```python
from build123d import *

# Parameters (mm, degrees)
BOSS_EXTRU_1_DEPTH      = 15
ESQUISSE3_W             = 30
ESQUISSE3_H             = 15
ENL_V_MAT_EXTRU_1_DEPTH = 15


with BuildPart() as part:
    # Esquisse2 → Boss.-Extru.1 (new body)
    with BuildSketch(Plane.XY):
        with BuildLine():
            Line((-120, 0), (120, 0))
            Line((120, 0), (120, 15))
            Line((120, 15), (120, 55.414518843))
            Line((120, 55.414518843), (120, 75.414518843))
            Line((120, 75.414518843), (120, 90))
            ThreePointArc((120, 90), (117.071067812, 97.071067812), (110, 100))
            Line((110, 100), (-110, 100))
            ThreePointArc((-110, 100), (-117.071067812, 97.071067812), (-120, 90))
            Line((-120, 90), (-120, 75.414518843))
            Line((-120, 75.414518843), (-120, 55.414518843))
            Line((-120, 55.414518843), (-120, 15))
            Line((-120, 15), (-120, 0))
        make_face()
    extrude(amount=BOSS_EXTRU_1_DEPTH)

    # Esquisse3 → Enlèv. mat.-Extru.1 (cut)
    with BuildSketch(Plane.XY.offset(15)):
        with Locations((-105, 7.5)):
            Rectangle(ESQUISSE3_W, ESQUISSE3_H)
        Polygon((-5, 31.515847226), (-5, 0), (5, 0), (5, 31.515847226), (12.5, 31.515847226), (12.5, 41.515847226), (5, 41.515847226), (5, 50), (-5, 50), (-5, 41.515847226), (-12.5, 41.515847226), (-12.5, 31.515847226), align=None)
        with Locations((105, 7.5)):
            Rectangle(ESQUISSE3_W, ESQUISSE3_H)
    extrude(amount=-ENL_V_MAT_EXTRU_1_DEPTH, mode=Mode.SUBTRACT)


solid = part.part
```
Input: part model. Units: mm. Frame: model coordinates. A direction names the side the tool comes from. Round coordinates to 2 decimals unless told otherwise and drop trailing zeros. Loops run counter-clockwise (first coordinate to the right, second up) from the corner with the lowest first, then second, coordinate; pieces in that order, holes last. Notation, with made-up numbers: M 56,-14.5 L 98,-14.5 A17 cw 98,1.5 Z; hole C 17,25.25 d6. An arc over 180 degrees is marked long. Answer in a Markdown table with one row per item. Add a question column.
1. Mould query, pull axis X, two halves, no side actions, for faces 1 (the face through (-90, 7, 8)), 2 (the face through (-5, 46, 8)), 3 (the face through (117.15, 96.99, 7.4)). Classes: released by +X, released by -X, zero draft, split by the parting line, or undercut.
2. Section A-A (z = 12). Output: boundary loops of the cut face in (x, y).
3. Set-up query: faces 4 (the face through (-12.5, 37, 8)), 5 (the face through (105, 15, 8)), 6 (the face through (5, 16, 8)), 7 (the face through (-105, 15, 8)). Return all of +Z, -Z, +X, -X, +Y, -Y with unobstructed straight access to the full face (end or side cutting, diameter ignored); none if empty.
4. Section B-B (x = -96). Output: boundary loops of the cut face in (y, z).
5. Contact query for flat-ended pins moving along their axis: pin 1 (3 mm diameter, centred on x = -2, z = 4.5, fed in from -Y); pin 2 (7.5 mm diameter, centred on x = 103, z = 9, fed in from -Y). Output: stop coordinate, or through.
6. Ray query, probe 1 along X at (y, z) = (17, 7.25); probe 2 along X at (y, z) = (6.5, 4.75); probe 3 along Y at (x, z) = (3, 1). Return the intervals inside material, ascending.
Values follow:
| question | item | result |
|---|---|---|
| 1 | face 1 | released by -X |
| 1 | face 2 | undercut |
| 1 | face 3 | released by +X |
| 2 | outline | M -120,15 L -90,15 L -90,0 L -5,0 L -5,31.52 L -12.5,31.52 L -12.5,41.52 L -5,41.52 L -5,50 L 5,50 L 5,41.52 L 12.5,41.52 L 12.5,31.52 L 5,31.52 L 5,0 L 90,0 L 90,15 L 120,15 L 120,90 A10 ccw 110,100 L -110,100 A10 ccw -120,90 Z |
| 3 | face 4 | +Z, -Z |
| 3 | face 5 | +Z, -Z, +X, -Y |
| 3 | face 6 | +Z, -Z, -Y |
| 3 | face 7 | +Z, -Z, -X, -Y |
| 4 | outline | M 15,0 L 100,0 L 100,15 L 15,15 Z |
| 5 | pin 1 | y = 50 |
| 5 | pin 2 | y = 15 |
| 6 | probe 1 | -120 to -5, 5 to 120 |
| 6 | probe 2 | -90 to -5, 5 to 90 |
| 6 | probe 3 | 50 to 100 |
